Source: CAD feature listing. Evaluate the final solid. Frame: model axes, mm. Face numbers are marked on the shaded views. Round coordinates to 2 decimals unless told otherwise and drop trailing zeros. Loops run counter-clockwise (first coordinate to the right, second up) from the corner with the lowest first, then second, coordinate; pieces in that order, holes last. Notation, with made-up numbers: M 35,55 L 53,55 A30 cw 53,86 Z; hole C 76.5,16.5 d3. An arc over 180 degrees is marked long. Answer as a JSON object with one key per item and string values.
from build123d import *

# Parameters (mm, degrees)
F0_R     = 11
F1_DEPTH = 8
F2_W     = 1
F2_H     = 1
F2_R     = 0.5
F3_DEPTH = 3


with BuildPart() as f1:
    # F0 (on Top) → F1 (new body)
    with BuildSketch(Plane.XY):
        with BuildLine():
            ThreePointArc((-8.5, 0), (0, 8.5), (8.5, 0))
            Line((8.5, 0), (46.5, 0))
            Line((46.5, 0), (27.5, 32.908965))
            ThreePointArc((27.5, 32.908965), (15.888784, 36.020181), (19, 47.631397))
            Line((19, 47.631397), (0, 80.540363))
            Line((0, 80.540363), (-19, 47.631397))
            ThreePointArc((-19, 47.631397), (-15.888784, 36.020181), (-27.5, 32.908965))
            Line((-27.5, 32.908965), (-46.5, 0))
            Line((-46.5, 0), (-8.5, 0))
        make_face()
        with Locations((-23.382686, 13.346788)):
            Circle(F0_R, mode=Mode.SUBTRACT)
        with Locations((23.382686, 13.346788)):
            Circle(F0_R, mode=Mode.SUBTRACT)
        with Locations((0, 26.846788)):
            Circle(F0_R, mode=Mode.SUBTRACT)
        with Locations((0, 53.846788)):
            Circle(F0_R, mode=Mode.SUBTRACT)
    extrude(amount=F1_DEPTH)

    # F2 (on face) → F3 (cut)
    with BuildSketch(Plane.XY.offset(8)):
        Polygon((-6.540234, 12), (-4.540234, 12), (-4.540234, 9), (-3.540234, 9), (-3.540234, 12), (-3.540234, 15), (-6.540234, 15), align=None)
        with Locations((-5.040234, 13.5)):
            Rectangle(F2_W, F2_H, mode=Mode.SUBTRACT)
        Polygon((2.449274, 14.999983), (-2.095626, 14.999983), (-2.095626, 13.999983), (0.904374, 13.999983), (-1.820119, 9), (-0.820119, 9), align=None)
        Polygon((2.912836, 9), (6.912836, 9), (6.912836, 10), (3.912836, 10), (3.912836, 11.5), (6.912836, 11.5), (6.912836, 14.999983), (2.857154, 14.999983), (2.857154, 13.999983), (5.857154, 13.999983), (5.912836, 12.5), (2.912836, 12.5), (2.912836, 11.5), align=None)
        Polygon((8.759619, 35.368257), (13.955771, 38.368257), (13.455771, 39.234283), (11.290708, 37.984283), (10.290708, 39.716334), (12.455771, 40.966334), (11.955771, 41.832359), (6.759619, 38.832359), (7.259619, 37.966334), (9.424682, 39.216334), (10.424682, 37.484283), (8.259619, 36.234283), align=None)
        with Locations((1.763236, 9.5)):
            Circle(F2_R)
        with Locations((15.022759, 35.520181)):
            Circle(F2_R)
        Polygon((12.759619, 28.440054), (17.955771, 31.440054), (16.455771, 34.03813), (15.589746, 33.53813), (16.589746, 31.80608), (12.259619, 29.30608), align=None)
    extrude(amount=-F3_DEPTH, mode=Mode.SUBTRACT)


solid = f1.part
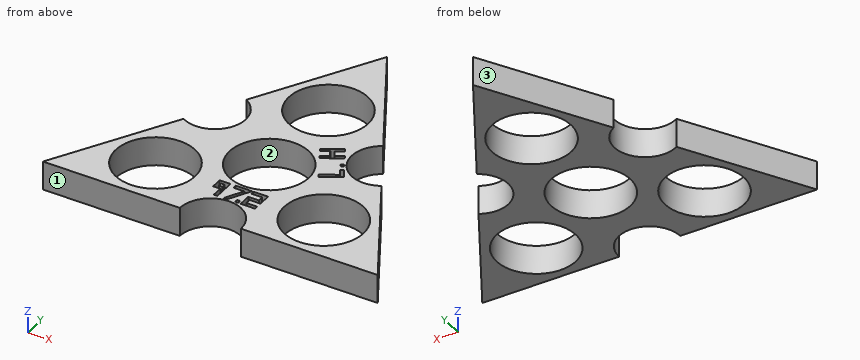
Item 1: Contact query for flat-ended pins moving along their axis: pin 1 Ø0.9 at (x, z) = (5, 6.5) entering from -Y; pin 2 Ø0.9 at (y, z) = (10, 6) entering from +X; pin 3 Ø0.5 at (x, z) = (-5, 6.5) entering from -Y; pin 4 Ø8 at (x, y) = (18, 14) entering from -Z. Output: stop coordinate, or through.
Answer sheet:
{"pin 1": "stops at y = 6.52", "pin 2": "stops at x = 40.99", "pin 3": "stops at y = 6.68", "pin 4": "passes through"}
Item 2: Section A-A on x = -32. Return the cut outline in (y, z), then the cut area to 3 significant figures.
Answer sheet:
{"outline": "M 0,0 L 6.51,0 L 6.51,8 L 0,8 Z; M 20.18,0 L 25.11,0 L 25.11,8 L 20.18,8 Z", "area": "91.5 mm²"}
Item 3: Section C-C on z = 3.5. Return the cut outline in (x, y).
Answer sheet:
{"outline": "M -46.5,0 L -8.5,0 A8.5 cw 8.5,0 L 46.5,0 L 27.5,32.91 A8.5 cw 19,47.63 L 0,80.54 L -19,47.63 A8.5 cw -27.5,32.91 Z; hole C -23.38,13.35 d22; hole C 0,26.85 d22; hole C 0,53.85 d22; hole C 23.38,13.35 d22"}
Item 4: Line query: probe 1 along X at (y, z) = (21, 4.75); probe 2 along X at (y, z) = (19, 1.5); probe 3 along Y at (x, z) = (-17.5, 7). Output: solid intervals per line, ascending. Write a range as from..to.
Answer sheet:
{"probe 1": "x = -34.38..-31.28, -15.48..-9.32, 9.32..15.48, 31.28..34.38", "probe 2": "x = -35.53..-32.82, -13.95..-7.71, 7.71..13.95, 32.82..35.53", "probe 3": "y = 0..4.05, 22.64..34.01, 46.53..50.23"}
Item 5: Pull-direction query (X, two-part tool) for the marked faces 1, 2 and 3; classes: pulls with the +X half, pulls with the -X half, needs draft (parallel to the pull), parting line crosses it, or undercut.
Answer sheet:
{"face 1": "needs draft", "face 2": "undercut", "face 3": "pulls with the -X half"}
Item 6: Section B-B on y = 7. Return the cut outline in (x, z).
Answer sheet:
{"outline": "M -42.46,0 L -32.37,0 L -32.37,8 L -42.46,8 Z; M -14.4,0 L -4.82,0 L -4.82,8 L -14.4,8 Z; M 4.82,0 L 14.4,0 L 14.4,8 L 4.82,8 Z; M 32.37,0 L 42.46,0 L 42.46,8 L 32.37,8 Z"}
Item 7: Section D-D on y = 44. Return the cut outline in (x, z), then the cut area to 3 significant figures.
Answer sheet:
{"outline": "M -15.61,0 L -4.9,0 L -4.9,8 L -15.61,8 Z; M 4.9,0 L 15.61,0 L 15.61,8 L 4.9,8 Z", "area": "171 mm²"}
